Can you work these out from the model? Positions are in its coordinate system, mm. Coordinates: 2 decimals unless noted, no trailing zeros. Loops run counter-clockwise (first coordinate to the right, second up) from the corner with the lowest first, then second, coordinate; pieces in that order, holes last.
```python
from build123d import *

# Parameters (mm, degrees)
MODEL_R                  = 6.5
MODEL_R_2                = 5.25
MODEL_W                  = 165
MODEL_H                  = 32
RESSALTO_EXTRUS_O1_DEPTH = 2


with BuildPart() as part:
    # Model → Ressalto-extrusão1 (new body)
    with BuildSketch(Plane.XY):
        Polygon((270.074227849, 25.427113901), (280.074227849, 25.427113901), (280.074227849, 35.427113901), (288.074227849, 35.427113901), (288.074227849, 173.427113901), (280.074227849, 173.427113901), (280.074227849, 183.427113901), (270.074227849, 183.427113901), (270.074227849, 191.427113901), (22.074227849, 191.427113901), (22.074227849, 183.427113901), (12.074227849, 183.427113901), (12.074227849, 173.427113901), (4.074227849, 173.427113901), (4.074227849, 35.427113901), (12.074227849, 35.427113901), (12.074227849, 25.427113901), (22.074227849, 25.427113901), (22.074227849, 17.427113901), (270.074227849, 17.427113901), align=None)
        with Locations((36.574227849, 160.927113901)):
            Circle(MODEL_R, mode=Mode.SUBTRACT)
        with Locations((36.574227849, 136.177113901)):
            Circle(MODEL_R, mode=Mode.SUBTRACT)
        with Locations((93.574227849, 110.927113901)):
            Circle(MODEL_R, mode=Mode.SUBTRACT)
        with Locations((144.574227849, 110.927113901)):
            Circle(MODEL_R, mode=Mode.SUBTRACT)
        with Locations((195.574227849, 110.927113901)):
            Circle(MODEL_R, mode=Mode.SUBTRACT)
        with Locations((195.574227849, 160.927113901)):
            Circle(MODEL_R, mode=Mode.SUBTRACT)
        with Locations((144.574227849, 160.927113901)):
            Circle(MODEL_R, mode=Mode.SUBTRACT)
        with Locations((93.574227849, 160.927113901)):
            Circle(MODEL_R, mode=Mode.SUBTRACT)
        with Locations((246.574227849, 142.427113901)):
            Circle(MODEL_R_2, mode=Mode.SUBTRACT)
        with Locations((259.574227849, 142.427113901)):
            Circle(MODEL_R_2, mode=Mode.SUBTRACT)
        with Locations((259.574227849, 129.427113901)):
            Circle(MODEL_R_2, mode=Mode.SUBTRACT)
        with Locations((246.574227849, 129.427113901)):
            Circle(MODEL_R_2, mode=Mode.SUBTRACT)
        with Locations((142.574227849, 136.177113901)):
            Rectangle(MODEL_W, MODEL_H, mode=Mode.SUBTRACT)
    extrude(amount=RESSALTO_EXTRUS_O1_DEPTH)


solid = part.part
```
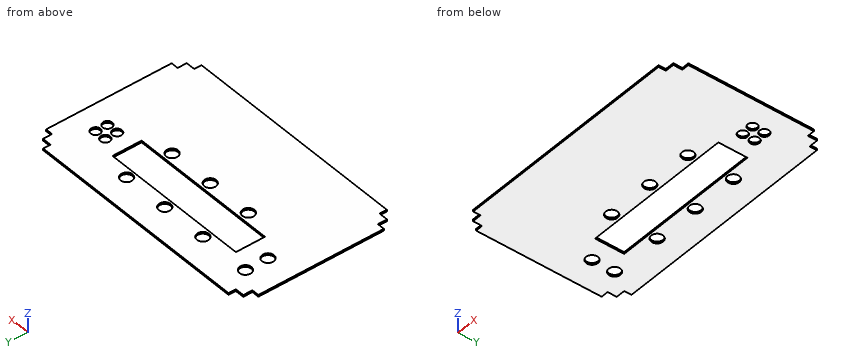
(1) If I drill on probe 1 along Y at (x, z) = (188, 0.95); probe 2 along X at (y, z) = (148.5, 0.75); probe 3 along Y at (x, z) = (200.5, 1.9), over which ranges is the centre line in solid material (lowest first)?
Check values:
probe 1: y = 17.43 to 120.18, 152.18 to 191.43
probe 2: x = 4.07 to 60.07, 225.07 to 288.07
probe 3: y = 17.43 to 106.69, 115.17 to 120.18, 152.18 to 156.69, 165.17 to 191.43
(2) I want a section at A-A on x = 76. Write out the boundary of the cut face in (y, z), then the cut area to 3 significant figures.
Check values:
outline: (17.43, 0) - (120.18, 0) - (120.18, 2) - (17.43, 2) - close; (152.18, 0) - (191.43, 0) - (191.43, 2) - (152.18, 2) - close
area: 284 mm2
(3) I want a section at B-B on y = 158. Write out the boundary of the cut face in (x, z), then the cut area to 3 significant figures.
Check values:
outline: (4.07, 0) - (30.77, 0) - (30.77, 2) - (4.07, 2) - close; (42.38, 0) - (87.77, 0) - (87.77, 2) - (42.38, 2) - close; (99.38, 0) - (138.77, 0) - (138.77, 2) - (99.38, 2) - close; (150.38, 0) - (189.77, 0) - (189.77, 2) - (150.38, 2) - close; (201.38, 0) - (288.07, 0) - (288.07, 2) - (201.38, 2) - close
area: 475 mm2
(4) I'm going to push flat-ended pins straight in: pin 1 (1 mm diameter, centred on x = 8.5, z = 1.5, fed in from -Y); pin 2 (1 mm diameter, centred on x = 276, z = 1.5, fed in from -Y); pin 3 (0.6 mm diameter, centred on x = 8.5, z = 1, fed in from +Y). Where does each tip first touch, or does it pass through?
Check values:
pin 1: stops at y = 35.43
pin 2: stops at y = 25.43
pin 3: stops at y = 173.43
(5) I want a section at C-C on x = 147. Write out the boundary of the cut face in (y, z).
Check values:
outline: (17.43, 0) - (104.9, 0) - (104.9, 2) - (17.43, 2) - close; (116.96, 0) - (120.18, 0) - (120.18, 2) - (116.96, 2) - close; (152.18, 0) - (154.9, 0) - (154.9, 2) - (152.18, 2) - close; (166.96, 0) - (191.43, 0) - (191.43, 2) - (166.96, 2) - close
(6) I want a section at D-D on z = 0.45. State how many separate pieces and enclosed holes the cut face has, then the cut area to 3 significant figures.
Check values:
separate pieces: 1
enclosed holes: 13
area: 41,800 mm2
